Part model, mm, in its own coordinate system. Face numbers are marked on the shaded views. A direction names the side the tool comes from. Coordinates: 2 decimals unless noted, no trailing zeros. Loops run counter-clockwise (first coordinate to the right, second up) from the corner with the lowest first, then second, coordinate; pieces in that order, holes last. Notation, with made-up numbers: M 4.5,69 L 46.5,69 A11 cw 46.5,81 Z; hole C -35,43 d8. An arc over 180 degrees is marked long. Answer as a JSON object with one key per item and string values. Group by question number.
1. Drop flat-ended pins along their axis: pin 1 Ø2 at (x, y) = (47.5, 29) entering from +Z; pin 2 Ø3 at (x, z) = (28.5, 7) entering from -Y; pin 3 Ø10 at (x, z) = (15, -3) entering from -Y. Give the stop position or say it passes through.
2. Mould opens along Y. For the marked faces 1, 2 and 3 say: released by +Y, released by -Y, zero draft, split by the parting line, or undercut.
3. Drill centre lines: L1, parallel to Y at x = 0, z = 0.5; L2, parallel to Y at x = 0, z = -8; L3, parallel to X at y = 29, z = -4.5. Where is each one in solid material? Low to high.
4. 3-axis set-ups, long thin cutter, end or side, ignore diameter. For the marked faces 4, 5 and 6: which of +Z, -Z, +X, -X, +Y, -Y reach the whole face in a straight line?
5. Saw through at B-B on z = -1. Write the cut outline in (x, y).
6. Saw through at C-C on x = 0. Count the separate pieces of the cut face and the enclosed holes in it, then the cut area to 3 significant figures.
7. Saw through at D-D on z = 9. Write the cut outline in (x, y), then the cut area to 3 significant figures.
8. Saw through at A-A on y = 0. Write the cut outline in (x, z).
from build123d import *

# Parameters (mm, degrees)
CUT_EXTRUDE1_DEPTH      = 96.530099969
CUT_EXTRUDE1_DEPTH_BACK = 96.530099969
SKETCH2_R               = 10


with BuildPart() as part:
    # Sketch1 → Revolve1 (revolve)
    with BuildSketch(Plane(origin=(0, 0, 0), x_dir=(0, 0, -1), z_dir=(1, 0, 0)), mode=Mode.PRIVATE) as revolve1_sk:
        Polygon((12.5, 65), (-12.5, 65), (-12.5, 60), (-6, 60), (-6, 41.964344451), (-6, 27.5), (-20, 20), (-20, 15), (20, 15), (20, 20), (6, 27.5), (6, 41.964344451), (6, 60), (12.5, 60), align=None)
    revolve(revolve1_sk.sketch.rotate(Axis((0, 0, -27.705838771), (0, 0, 1)), 90), axis=Axis((0, 0, -27.705838771), (0, 0, 1)))

    # Sketch2 → Cut-Extrude1 (cut, two sides: drawn at the far end of the back side and taken through both)
    with BuildSketch(Plane.XY.offset(6).offset(-CUT_EXTRUDE1_DEPTH_BACK)):
        with Locations((0, 42)):
            Circle(SKETCH2_R)
        with Locations((36.373066959, 21)):
            Circle(SKETCH2_R)
        with Locations((36.373066959, -21)):
            Circle(SKETCH2_R)
        with Locations((0, -42)):
            Circle(SKETCH2_R)
        with Locations((-36.373066959, -21)):
            Circle(SKETCH2_R)
        with Locations((-36.373066959, 21)):
            Circle(SKETCH2_R)
    extrude(amount=CUT_EXTRUDE1_DEPTH + CUT_EXTRUDE1_DEPTH_BACK, mode=Mode.SUBTRACT)


solid = part.part
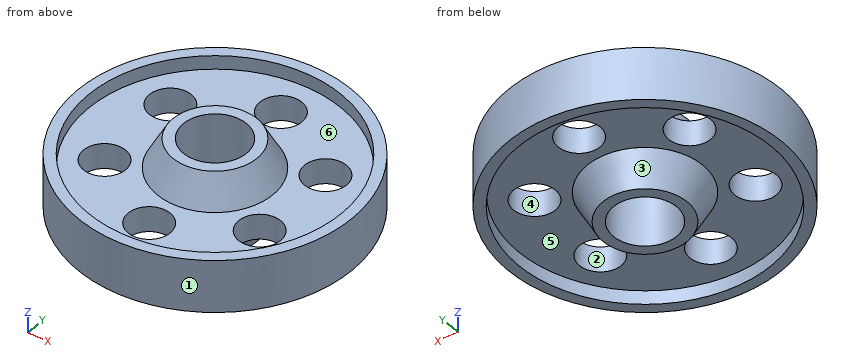
Outcome:
{
 "1": {"pin 1": "stops at z = 6", "pin 2": "stops at y = -59.13", "pin 3": "stops at y = -64.23"},
 "2": {"face 1": "split by the parting line", "face 2": "undercut", "face 3": "undercut"},
 "3": {"L1": "y = -65 to -52, -32 to -15, 15 to 32, 52 to 65", "L2": "y = -65 to -60, -26.43 to -15, 15 to 26.43, 60 to 65", "L3": "x = -58.17 to -42.37, -30.37 to 30.37, 42.37 to 58.17"},
 "4": {"face 4": "+Z, -Z", "face 5": "-Z", "face 6": "+Z"},
 "5": {"outline": "C 0,0 d130; hole C -36.37,-21 d20; hole C -36.37,21 d20; hole C 0,0 d30; hole C 0,-42 d20; hole C 0,42 d20; hole C 36.37,-21 d20; hole C 36.37,21 d20"},
 "6": {"separate pieces": "4", "enclosed holes": "0", "area": "1,340 mm²"},
 "7": {"outline": "C 0,0 d130; C 0,0 d51.79; hole C 0,0 d120; hole C 0,0 d30", "area": "3,360 mm²"},
 "8": {"outline": "M -65,-12.5 L -60,-12.5 L -60,-6 L -27.5,-6 L -20,-20 L -15,-20 L -15,20 L -20,20 L -27.5,6 L -60,6 L -60,12.5 L -65,12.5 Z; M 15,-20 L 20,-20 L 27.5,-6 L 60,-6 L 60,-12.5 L 65,-12.5 L 65,12.5 L 60,12.5 L 60,6 L 27.5,6 L 20,20 L 15,20 Z"}
}
